Input: part model. Units: mm. Frame: model coordinates. Face numbers are marked on the shaded views. Give positions to 0.01 mm unless a question says otherwise; leave off trailing zeros. Loops run counter-clockwise (first coordinate to the right, second up) from the corner with the lowest first, then second, coordinate; pieces in that order, holes last. Notation, with made-up numbers: (27, 25) -> (38, 25) arc R23 cw to (38, 46) -> close; hole circle Ø1 at (36, 67). An arc over 180 degrees is marked (long way). One line per question, with ' | ' between items.
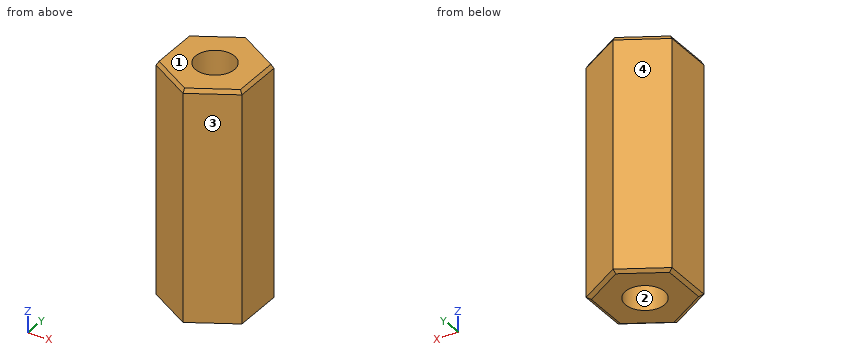
from build123d import *
from OCP.BRepFilletAPI import BRepFilletAPI_MakeChamfer

# Parameters (mm, degrees)
EXTRUDE_1_DEPTH    = 7.5
HOLE_WIZARD_M3_1_D = 2.5
CHAMFER_2_SIZE     = 0.25
CHAMFER_2_SIZE2    = 0.144337567


with BuildPart() as part:
    # ｽｹｯﾁ1 → ﾎﾞｽ - 押し出し1 (new, symmetric)
    with BuildSketch(Plane.XY):
        Polygon((-2.75, 1.58771324), (-2.75, -1.58771324), (0, -3.175426481), (2.75, -1.58771324), (2.75, 1.58771324), (0, 3.175426481), align=None)
    extrude(amount=EXTRUDE_1_DEPTH, both=True)

    # M3 ねじ穴1 (through all)
    with Locations(Plane.XY.offset(7.5)):
        with Locations((0, 0)):
            Hole(HOLE_WIZARD_M3_1_D / 2)

    # 面取り2: one chamfer whose edges measure the first distance from different faces: ONE call of the kernel's chamfer builder (chamfer() names one face for all edges)
    chamfer_2_edges_1 = [part.edges().sort_by_distance(p)[0] for p in [
        (-1.375, -2.38156986, 7.5),
    ]]
    chamfer_2_side_1 = [part.faces().sort_by_distance(p)[0] for p in [
        (-1.375, -2.38156986, 0),
    ]]
    chamfer_2_edges_2 = [part.edges().sort_by_distance(p)[0] for p in [
        (1.375, -2.38156986, 7.5),
    ]]
    chamfer_2_side_2 = [part.faces().sort_by_distance(p)[0] for p in [
        (1.375, -2.38156986, 0),
    ]]
    chamfer_2_edges_3 = [part.edges().sort_by_distance(p)[0] for p in [
        (2.75, 0, 7.5),
    ]]
    chamfer_2_side_3 = [part.faces().sort_by_distance(p)[0] for p in [
        (2.75, 0, 0),
    ]]
    chamfer_2_edges_4 = [part.edges().sort_by_distance(p)[0] for p in [
        (1.375, 2.38156986, 7.5),
    ]]
    chamfer_2_side_4 = [part.faces().sort_by_distance(p)[0] for p in [
        (1.375, 2.38156986, 0),
    ]]
    chamfer_2_edges_5 = [part.edges().sort_by_distance(p)[0] for p in [
        (-1.375, 2.38156986, 7.5),
    ]]
    chamfer_2_side_5 = [part.faces().sort_by_distance(p)[0] for p in [
        (-1.375, 2.38156986, 0),
    ]]
    chamfer_2_edges_6 = [part.edges().sort_by_distance(p)[0] for p in [
        (1.375, 2.38156986, -7.5),
        (2.75, 0, -7.5),
        (1.375, -2.38156986, -7.5),
        (-1.375, -2.38156986, -7.5),
        (-2.75, 0, -7.5),
        (-1.375, 2.38156986, -7.5),
    ]]
    chamfer_2_side_6 = [part.faces().sort_by_distance(p)[0] for p in [
        (-2.665986112, 0, -7.5),
    ]]
    chamfer_2_edges_7 = [part.edges().sort_by_distance(p)[0] for p in [
        (-2.75, 0, 7.5),
    ]]
    chamfer_2_side_7 = [part.faces().sort_by_distance(p)[0] for p in [
        (-2.75, 0, 0),
    ]]
    chamfer_2 = BRepFilletAPI_MakeChamfer(part.part.solid().wrapped)
    for e in chamfer_2_edges_1:
        chamfer_2.Add(CHAMFER_2_SIZE, CHAMFER_2_SIZE2, e.wrapped, chamfer_2_side_1[0].wrapped)  # the first distance lies on this face
    for e in chamfer_2_edges_2:
        chamfer_2.Add(CHAMFER_2_SIZE, CHAMFER_2_SIZE2, e.wrapped, chamfer_2_side_2[0].wrapped)  # the first distance lies on this face
    for e in chamfer_2_edges_3:
        chamfer_2.Add(CHAMFER_2_SIZE, CHAMFER_2_SIZE2, e.wrapped, chamfer_2_side_3[0].wrapped)  # the first distance lies on this face
    for e in chamfer_2_edges_4:
        chamfer_2.Add(CHAMFER_2_SIZE, CHAMFER_2_SIZE2, e.wrapped, chamfer_2_side_4[0].wrapped)  # the first distance lies on this face
    for e in chamfer_2_edges_5:
        chamfer_2.Add(CHAMFER_2_SIZE, CHAMFER_2_SIZE2, e.wrapped, chamfer_2_side_5[0].wrapped)  # the first distance lies on this face
    for e in chamfer_2_edges_6:
        chamfer_2.Add(CHAMFER_2_SIZE, CHAMFER_2_SIZE2, e.wrapped, chamfer_2_side_6[0].wrapped)  # the first distance lies on this face
    for e in chamfer_2_edges_7:
        chamfer_2.Add(CHAMFER_2_SIZE, CHAMFER_2_SIZE2, e.wrapped, chamfer_2_side_7[0].wrapped)  # the first distance lies on this face
    add(Compound.cast(chamfer_2.Shape()), mode=Mode.REPLACE)


solid = part.part
1. Pull-direction query (Y, two-part tool) for the marked faces 1, 2, 3 and 4; classes: pulls with the +Y half, pulls with the -Y half, needs draft (parallel to the pull), parting line crosses it, or undercut.
Determined:
face 1: needs draft | face 2: undercut | face 3: pulls with the -Y half | face 4: pulls with the +Y half
2. Section query D-D (x = -2.3). Output: boundary loops of the cut face in (y, z), then the cut area to 3 significant figures.
Determined:
outline: (-1.85, -7.36) -> (-1.56, -7.5) -> (1.56, -7.5) -> (1.85, -7.36) -> (1.85, 7.25) -> (1.68, 7.5) -> (-1.68, 7.5) -> (-1.85, 7.25) -> close | area: 55.3 mm2
3. Section query A-A (z = 1). Output: boundary loops of the cut face in (x, y), then the cut area to 3 significant figures.
Determined:
outline: (-2.75, -1.59) -> (0, -3.18) -> (2.75, -1.59) -> (2.75, 1.59) -> (0, 3.18) -> (-2.75, 1.59) -> close; hole circle Ø2.5 at (0, 0) | area: 21.3 mm2
4. Ray query, line 1 along X through (y, z) = (1, 4); line 2 along Y through (x, z) = (-0.05, -6). Return the intervals inside material, ascending. Write a range as from..to.
Determined:
line 1: x = -2.75..-0.75, 0.75..2.75 | line 2: y = -3.15..-1.25, 1.25..3.15
5. Section query C-C (x = -0.7). Output: boundary loops of the cut face in (y, z).
Determined:
outline: (-2.77, -7.36) -> (-2.48, -7.5) -> (-1.04, -7.5) -> (-1.04, 7.5) -> (-2.6, 7.5) -> (-2.77, 7.25) -> close; (1.04, -7.5) -> (2.48, -7.5) -> (2.77, -7.36) -> (2.77, 7.25) -> (2.6, 7.5) -> (1.04, 7.5) -> close
6. Pin query (flat end, axial travel): P1, Ø1.5, axis at x = 0, y = 0, coming from the +Z side. Return the tip coordinate at first contact, or that it passes through.
Determined:
P1: passes through
7. Section query B-B (y = 0). Output: boundary loops of the cut face in (x, z).
Determined:
outline: (-2.75, -7.36) -> (-2.5, -7.5) -> (-1.25, -7.5) -> (-1.25, 7.5) -> (-2.61, 7.5) -> (-2.75, 7.25) -> close; (1.25, -7.5) -> (2.5, -7.5) -> (2.75, -7.36) -> (2.75, 7.25) -> (2.61, 7.5) -> (1.25, 7.5) -> close
